Here's the drawing with two shaded views (mm, measured from the low corner). I have some questions. A direction names the side the tool comes from. Give positions to 0.01 mm unless a question says otherwise; leave off trailing zeros. Loops run counter-clockwise (first coordinate to the right, second up) from the corner with the lowest first, then second, coordinate; pieces in that order, holes last. Notation, with made-up numbers: (30, -4) - (50, -4) arc R24 cw to (50, 25) - close; hole circle Ø7 at (14.5, 43). An arc over 180 degrees is marked (long way). Write each question's results on one line, items separated by ' | '. Start each with the question number.
1) I want a section at A-A, the plane y = 33. Write out the boundary of the cut face in (x, z), and give its area (3 significant figures).
2) I want a section at C-C, the plane z = 6.75. Count the separate pieces of the cut face and the enclosed holes in it, and give its area (3 significant figures).
3) If we mould it in two halves opening along X, with no side actions, what happens to the marked faces 1, 2, 3 and 4? For each: +X half, -X half, draft (parallel to the pull), parting line (faces both ways), or undercut.
4) On a 3-axis mill with a long thin cutter (end or side, diameter ignored), from which of +Z, -Z, +X, -X, +Y, -Y can I reach the whole of each face in a straight line? I mean the marked faces 5, 6 and 7. Say none if no direction works.
5) If I drill on probe 1 along Y at (x, z) = (43, 15); probe 2 along X at (y, z) = (20, 6); probe 3 along Y at (x, z) = (30, 10.75), over which ranges is the centre line in solid material (lowest first)? Write a range as [from, to].
6) I'm going to push flat-ended pins straight in: pin 1 (7 mm diameter, centred on x = 20, z = 17.5, fed in from -Y); pin 2 (3 mm diameter, centred on x = 2, y = 49, fed in from -Z); pin 3 (12 mm diameter, centred on x = 34.5, z = 18, fed in from +Y). Where does each tip first touch, or does it pass through?
7) I want a section at B-B, the plane x = 26.5. Write out the boundary of the cut face in (y, z).
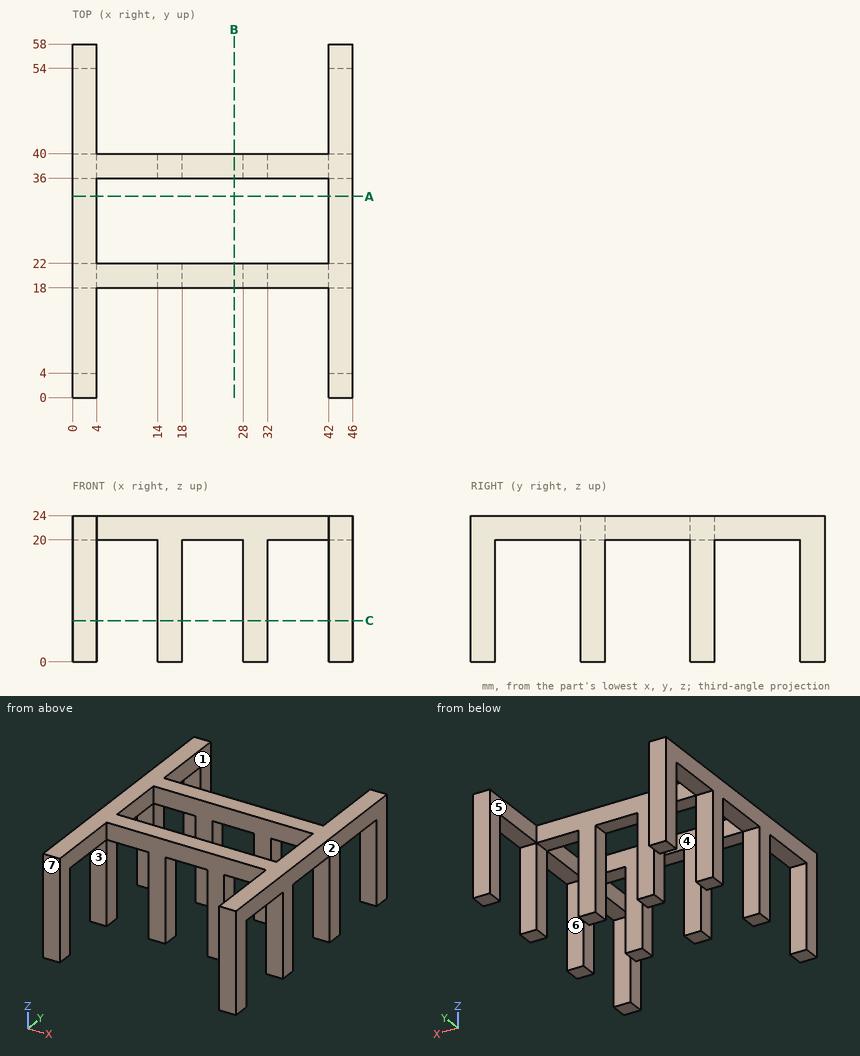
Answers:
1) outline: (0, 20) - (4, 20) - (4, 24) - (0, 24) - close; (42, 20) - (46, 20) - (46, 24) - (42, 24) - close | area: 32.0 mm2
2) separate pieces: 12 | enclosed holes: 0 | area: 192 mm2
3) face 1: undercut | face 2: +X half | face 3: draft | face 4: undercut
4) face 5: +Z, -Z, +Y | face 6: -Z, +X, -X | face 7: +Z, -Z, +X, -X, -Y
5) probe 1: y = [0, 4], [18, 22], [36, 40], [54, 58] | probe 2: x = [0, 4], [14, 18], [28, 32], [42, 46] | probe 3: y = [18, 22], [36, 40]
6) pin 1: stops at y = 18 | pin 2: stops at z = 20 | pin 3: stops at y = 40
7) outline: (18, 20) - (22, 20) - (22, 24) - (18, 24) - close; (36, 20) - (40, 20) - (40, 24) - (36, 24) - close
